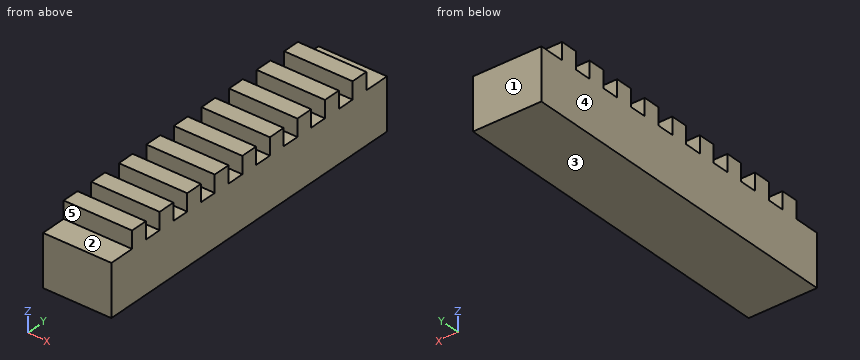
```python
from build123d import *

# Parameters (mm, degrees)
SKETCH1_W           = 20
SKETCH1_H           = 100
BOSS_EXTRUDE1_DEPTH = 15
SKETCH2_W           = 20
SKETCH2_H           = 5
BOSS_EXTRUDE2_DEPTH = 5


with BuildPart() as part:
    # Sketch1 → Boss-Extrude1 (new body)
    with BuildSketch(Plane.XY):
        Rectangle(SKETCH1_W, SKETCH1_H)
    extrude(amount=BOSS_EXTRUDE1_DEPTH)

    # Sketch2 → Boss-Extrude2 (add)
    with BuildSketch(Plane.XY.offset(15)):
        Rectangle(SKETCH2_W, SKETCH2_H)
        with Locations((0, -10)):
            Rectangle(SKETCH2_W, SKETCH2_H)
        with Locations((0, -20)):
            Rectangle(SKETCH2_W, SKETCH2_H)
        with Locations((0, -30)):
            Rectangle(SKETCH2_W, SKETCH2_H)
        with Locations((0, -40)):
            Rectangle(SKETCH2_W, SKETCH2_H)
        with Locations((0, 10)):
            Rectangle(SKETCH2_W, SKETCH2_H)
        with Locations((0, 20)):
            Rectangle(SKETCH2_W, SKETCH2_H)
        with Locations((0, 30)):
            Rectangle(SKETCH2_W, SKETCH2_H)
        with Locations((0, 40)):
            Rectangle(SKETCH2_W, SKETCH2_H)
    extrude(amount=BOSS_EXTRUDE2_DEPTH)


solid = part.part
```
Input: part model. Units: mm. Frame: model coordinates. Face numbers are marked on the shaded views. A direction names the side the tool comes from. Coordinates: 2 decimals unless noted, no trailing zeros. Write each loop counter-clockwise with the first axis right and the second up, starting at its lowest first coordinate (ties: lowest second). Pieces come first, ordered by that corner, then holes. Notation, with made-up numbers: (68, 86) -> (80, 86) arc R24 cw to (80, 115) -> close; hole circle Ø11 at (-30.5, 64). An arc over 180 degrees is marked (long way). Answer as a JSON object with one key per item and string values.
1. Access query for the marked faces 4 and 5. Directions: +Z, -Z, +X, -X, +Y, -Y. A direction counts if a zero-diameter tool reaches every point of the face in a straight line with its end or side. Return the directions, or none.
Result set:
{"face 4": "+Z, -Z, -X, +Y, -Y", "face 5": "+Z, +X, -X, -Y"}
2. Material intervals for line 1 (Z direction, x = 2.25, y = 16), sorted ascending. Write a range as from..to.
Result set:
{"line 1": "z = 0..15"}
3. First-contact query: P1, Ø4, axis at x = -0.5, z = 17.5, coming from the +Y side; P2, Ø1.5, axis at x = 4.5, y = -36, coming from the +Z side; P3, Ø1.5, axis at x = 0.5, z = 16.5, coming from the -Y side. Flat tips, straight axial feed; report the tip coordinate or a pass-through.
Result set:
{"P1": "stops at y = 42.5", "P2": "stops at z = 15", "P3": "stops at y = -42.5"}
4. Section A-A on y = 13.5. Return the cut outline in (x, z), then the cut area to 3 significant figures.
Result set:
{"outline": "(-10, 0) -> (10, 0) -> (10, 15) -> (-10, 15) -> close", "area": "300 mm2"}
5. Mould query, pull axis Z, two halves, no side actions, for the marked faces 1, 2 and 3. Classes: released by +Z, released by -Z, zero draft, split by the parting line, or undercut.
Result set:
{"face 1": "zero draft", "face 2": "released by +Z", "face 3": "released by -Z"}
